from build123d import *

# Parameters (mm, degrees)
F0_R          = 5
F1_DEPTH      = 8
F3_DEPTH      = 9.906
F4_R          = 7
F5_DEPTH      = 10.001
F5_DEPTH_BACK = 10.001
F6_R          = 7
F6_R_2        = 5
F7_DEPTH      = 13.97
F7_DEPTH_BACK = 10.0076


with BuildPart() as f1:
    # F0 (on Top) → F1 (new body)
    with BuildSketch(Plane.XY):
        with BuildLine():
            Line((-19, -10), (19, -10))
            ThreePointArc((19, -10), (29, 0), (19, 10))
            Line((19, 10), (-19, 10))
            ThreePointArc((-19, 10), (-29, 0), (-19, -10))
        make_face()
        with Locations((-19, 0)):
            Circle(F0_R, mode=Mode.SUBTRACT)
        with Locations((19, 0)):
            Circle(F0_R, mode=Mode.SUBTRACT)
    extrude(amount=F1_DEPTH)

    # F2 (on Front) → F3 (join, symmetric)
    with BuildSketch(Plane.XZ):
        with BuildLine():
            Line((10, 0), (10, 11))
            ThreePointArc((10, 11), (0, 21), (-10, 11))
            Line((-10, 11), (-10, 0))
            Line((-10, 0), (10, 0))
        make_face()
    extrude(amount=F3_DEPTH, both=True)

    # F4 (on Front) → F5 (cut, two sides)
    with BuildSketch(Plane.XZ) as f5_sk:
        with Locations((0, 11)):
            Circle(F4_R)
    extrude(amount=F5_DEPTH, mode=Mode.SUBTRACT)
    extrude(f5_sk.sketch, amount=-F5_DEPTH_BACK, mode=Mode.SUBTRACT)

    # F6 (on Front) → F7 (join, two sides)
    with BuildSketch(Plane.XZ) as f7_sk:
        with Locations((0, 11)):
            Circle(F6_R)
        with Locations((0, 11)):
            Circle(F6_R_2, mode=Mode.SUBTRACT)
    extrude(amount=F7_DEPTH)
    extrude(f7_sk.sketch, amount=-F7_DEPTH_BACK)


solid = f1.part
Check sheet for the modelled part. Datum: model origin and axes. Units: mm. A direction names the side the tool comes from. Coordinates: 2 decimals unless noted, no trailing zeros. Write each loop counter-clockwise with the first axis right and the second up, starting at its lowest first coordinate (ties: lowest second). Pieces come first, ordered by that corner, then holes. Notation, with made-up numbers: M -36.5,-6.75 L -20.5,-6.75 A20 ccw -20.5,-0.75 Z; hole C 84.25,-9.5 d3. An arc over 180 degrees is marked long. Answer as CSV lines item,"result".
Q1. Mould release check, pull along X, two halves, no side actions. Record for faces 4 (the face through (-10, 0, 10)), 5 (the face through (-24, 0, 4)), 6 (the face through (-15, -4, 8)), 7 (the face through (10, 0, 9)): released by +X, released by -X, zero draft, split by the parting line, or undercut.
Check result:
face 4,"released by -X"
face 5,"undercut"
face 6,"zero draft"
face 7,"released by +X"
Q2. Material ranges on probe 1 along Y at (x, z) = (19, 5.5); probe 2 along Z at (x, y) = (0, 3); probe 3 along X at (y, z) = (-4.5, 7.25), recorded low to high. Write a range as from..to.
Check result:
probe 1,"-10..-5, 5..10"
probe 2,"0..6, 16..21"
probe 3,"-27.93..-21.18, -16.82..-3.31, 3.31..16.82, 21.18..27.93"
Q3. Go/stop test with flat-tipped pins: pin 1 (10 mm diameter, centred on x = -16.5, y = -3.5, fed in from +Z); pin 2 (2.5 mm diameter, centred on y = -1, z = 10, fed in from -X); pin 3 (6 mm diameter, centred on y = 3.5, z = 7, fed in from -X); pin 4 (6 mm diameter, centred on x = -19, y = 0, fed in from +Z). Record where each tip stops, or that it passes through.
Check result:
pin 1,"z = 8"
pin 2,"x = -10"
pin 3,"x = -28.99"
pin 4,"through"
Q4. Cross-section at A-A (z = 7.25). Count the separate pieces of the cut face and the enclosed holes in it, then the cut area to 3 significant figures.
Check result:
separate pieces,"2"
enclosed holes,"2"
area,"806 mm^2"
Q5. Cross-section at D-D (y = -9). Record the boundary of the cut face in (x, z).
Check result:
outline,"M -23.36,0 L 23.36,0 L 23.36,8 L 10,8 L 10,11 A10 ccw -10,11 L -10,8 L -23.36,8 Z; hole C 0,11 d10"
Q6. Cross-section at B-B (y = -6.5). Record the boundary of the cut face in (x, z), then the cut area to 3 significant figures.
Check result:
outline,"M -26.6,0 L 26.6,0 L 26.6,8 L 10,8 L 10,11 A10 ccw -10,11 L -10,8 L -26.6,8 Z; hole C 0,11 d10"
area,"564 mm^2"
Q7. Set-up check for faces 1 (the face through (29, 0, 4)), 2 (the face through (-1.517, -11.91, 4.166)), 3 (the face through (0, -10, 3)): record each of +Z, -Z, +X, -X, +Y, -Y from which the full face is reachable in a straight line by a thin tool's end or side.
Check result:
face 1,"+Z, -Z, +X"
face 2,"-Y"
face 3,"-Z, -Y"
